Read the model definition and answer for the solid it produces. Units are mm, in the model's axes. Coordinates: 2 decimals unless noted, no trailing zeros. Loops run counter-clockwise (first coordinate to the right, second up) from the corner with the lowest first, then second, coordinate; pieces in that order, holes last. Notation, with made-up numbers: M -26.5,77 L -17.5,77 A5 cw -17.5,81 Z; hole C -26,63 d6. An arc over 180 degrees is marked long. One line per item, written item: value. Start each with the question number.
```python
from build123d import *

# Parameters (mm, degrees)
SKETCH1_W           = 120
SKETCH1_H           = 140
BOSS_EXTRUDE1_DEPTH = 3
SKETCH2_R           = 1.5
CUT_EXTRUDE1_DEPTH  = 107.343782141
SKETCH3_R           = 1.5
CUT_EXTRUDE3_DEPTH  = 107.343782141
SKETCH4_R           = 1.5
CUT_EXTRUDE4_DEPTH  = 107.343782141
SKETCH5_R           = 1.5
CUT_EXTRUDE5_DEPTH  = 3
SKETCH6_R           = 1.525
SKETCH6_W           = 10
SKETCH6_H           = 2.05
SKETCH6_W_2         = 20
CUT_EXTRUDE7_DEPTH  = 107.343782141
SKETCH9_R           = 1.525
CUT_EXTRUDE8_DEPTH  = 3
SKETCH10_W          = 50
SKETCH10_H          = 15
CUT_EXTRUDE9_DEPTH  = 5
SKETCH11_R          = 1.5
CUT_EXTRUDE10_DEPTH = 5
SKETCH12_W          = 2.05
SKETCH12_H          = 20
CUT_EXTRUDE11_DEPTH = 10


with BuildPart() as part:
    # Sketch1 → Boss-Extrude1 (new body)
    with BuildSketch(Plane(origin=(0, 0, 0), x_dir=(1, 0, 0), z_dir=(0, 1, 0))):
        Rectangle(SKETCH1_W, SKETCH1_H)
        Polygon((-80, 21.791828604), (-60, 10), (-60, 70), (-80, 70), align=None)
        Polygon((80, 70), (60, 70), (60, 10), (80, 21.791828604), align=None)
    extrude(amount=BOSS_EXTRUDE1_DEPTH)

    # Sketch2 → Cut-Extrude1 (cut, through all)
    with BuildSketch(Plane(origin=(0, 3, 0), x_dir=(1, 0, 0), z_dir=(0, 1, 0))):
        with Locations(Location((28, -60, 0), (0, 0, 270))):
            Circle(SKETCH2_R)
        with Locations(Location((40.6, -26.277010809, 0), (0, 0, 270))):
            Circle(SKETCH2_R)
        with Locations(Location((-50, -55, 0), (0, 0, 270))):
            Circle(SKETCH2_R)
        with Locations(Location((8, -55, 0), (0, 0, 270))):
            Circle(SKETCH2_R)
        with Locations(Location((-50, -28.6, 0), (0, 0, 270))):
            Circle(SKETCH2_R)
        with Locations(Location((8, -28.6, 0), (0, 0, 270))):
            Circle(SKETCH2_R)
    extrude(amount=-CUT_EXTRUDE1_DEPTH, mode=Mode.SUBTRACT)

    # Sketch3 → Cut-Extrude3 (cut, through all)
    with BuildSketch(Plane(origin=(0, 3, 0), x_dir=(1, 0, 0), z_dir=(0, 1, 0))):
        with Locations(Location((-26.529579069, 61.385555627, 0), (0, 0, 270))):
            Circle(SKETCH3_R)
        with Locations(Location((-26.529579069, 6.385555627, 0), (0, 0, 90))):
            Circle(SKETCH3_R)
        with Locations(Location((26.470420931, 6.385555627, 0), (0, 0, 270))):
            Circle(SKETCH3_R)
        with Locations(Location((26.470420931, 61.385555627, 0), (0, 0, 90))):
            Circle(SKETCH3_R)
    extrude(amount=-CUT_EXTRUDE3_DEPTH, mode=Mode.SUBTRACT)

    # Sketch4 → Cut-Extrude4 (cut, through all)
    with BuildSketch(Plane(origin=(0, 3, 0), x_dir=(1, 0, 0), z_dir=(0, 1, 0))):
        with Locations(Location((-75, 34.863883517, 0), (0, 0, 270))):
            Circle(SKETCH4_R)
        with Locations(Location((-75, 58.863883517, 0), (0, 0, 270))):
            Circle(SKETCH4_R)
        with Locations(Location((-46, 34.863883517, 0), (0, 0, 90))):
            Circle(SKETCH4_R)
        with Locations(Location((-46, 58.863883517, 0), (0, 0, 90))):
            Circle(SKETCH4_R)
        with Locations(Location((46, 58.863883517, 0), (0, 0, 270))):
            Circle(SKETCH4_R)
        with Locations(Location((46, 34.863883517, 0), (0, 0, 270))):
            Circle(SKETCH4_R)
        with Locations(Location((75, 34.863883517, 0), (0, 0, 90))):
            Circle(SKETCH4_R)
        with Locations(Location((75, 58.863883517, 0), (0, 0, 90))):
            Circle(SKETCH4_R)
    extrude(amount=-CUT_EXTRUDE4_DEPTH, mode=Mode.SUBTRACT)

    # Sketch5 → Cut-Extrude5 (cut)
    with BuildSketch(Plane(origin=(0, 3, 0), x_dir=(1, 0, 0), z_dir=(0, 1, 0))):
        with Locations(Location((-68, 30, 0), (0, 0, 270))):
            Circle(SKETCH5_R)
        with Locations(Location((-53, 30, 0), (0, 0, 270))):
            Circle(SKETCH5_R)
    extrude(amount=-CUT_EXTRUDE5_DEPTH, mode=Mode.SUBTRACT)

    # Sketch6 → Cut-Extrude7 (cut, through all)
    with BuildSketch(Plane(origin=(0, 3, 0), x_dir=(1, 0, 0), z_dir=(0, 1, 0))):
        with Locations(Location((-53, -64.8, 0), (0, 0, 270))):
            Circle(SKETCH6_R)
        with Locations(Location((53, -64.8, 0), (0, 0, 90))):
            Circle(SKETCH6_R)
        with Locations((-40, -53.975)):
            Rectangle(SKETCH6_W, SKETCH6_H)
        with Locations((40, -53.975)):
            Rectangle(SKETCH6_W, SKETCH6_H)
        with Locations((30, -21.725)):
            Rectangle(SKETCH6_W_2, SKETCH6_H)
        with Locations((-30, -21.725)):
            Rectangle(SKETCH6_W_2, SKETCH6_H)
        with Locations((35, 23.325)):
            Rectangle(SKETCH6_W, SKETCH6_H)
        with Locations((-35, 23.325)):
            Rectangle(SKETCH6_W, SKETCH6_H)
    extrude(amount=-CUT_EXTRUDE7_DEPTH, mode=Mode.SUBTRACT)

    # Sketch9 → Cut-Extrude8 (cut)
    with BuildSketch(Plane(origin=(0, 3, 0), x_dir=(1, 0, 0), z_dir=(0, 1, 0))):
        with Locations(Location((-54, 22, 0), (0, 0, 270))):
            Circle(SKETCH9_R)
        with Locations(Location((54, 22, 0), (0, 0, 90))):
            Circle(SKETCH9_R)
    extrude(amount=-CUT_EXTRUDE8_DEPTH, mode=Mode.SUBTRACT)

    # Sketch10 → Cut-Extrude9 (cut)
    with BuildSketch(Plane(origin=(0, 3, 0), x_dir=(1, 0, 0), z_dir=(0, 1, 0))):
        with Locations((-0.2, -8.475074484)):
            Rectangle(SKETCH10_W, SKETCH10_H)
    extrude(amount=-CUT_EXTRUDE9_DEPTH, mode=Mode.SUBTRACT)

    # Sketch11 → Cut-Extrude10 (cut)
    with BuildSketch(Plane(origin=(0, 3, 0), x_dir=(1, 0, 0), z_dir=(0, 1, 0))):
        with Locations(Location((-53, 64, 0), (0, 0, 270))):
            Circle(SKETCH11_R)
        with Locations(Location((53, 64, 0), (0, 0, 270))):
            Circle(SKETCH11_R)
    extrude(amount=-CUT_EXTRUDE10_DEPTH, mode=Mode.SUBTRACT)

    # Sketch12 → Cut-Extrude11 (cut)
    with BuildSketch(Plane(origin=(0, 3, 0), x_dir=(1, 0, 0), z_dir=(0, 1, 0))):
        with Locations((-55.975, -15)):
            Rectangle(SKETCH12_W, SKETCH12_H)
        with Locations((55.975, -15)):
            Rectangle(SKETCH12_W, SKETCH12_H)
    extrude(amount=-CUT_EXTRUDE11_DEPTH, mode=Mode.SUBTRACT)


solid = part.part
```
1) Flat-ended cylindrical pins translate along their axes: pin 1 (1.5 mm diameter, centred on y = 2, z = 12, fed in from +X); pin 2 (2.5 mm diameter, centred on x = 28, z = 60, fed in from +Y). Find the tip coordinate at first contact, or state that the pin passes through.
2) Consider line 1 along X through (y, z) = (0.3, -6.5); line 2 along X through (y, z) = (1.5, -30); line 3 along Z through (x, y) = (-46, 0.85). Determine where each line is inside the solid, lowest interval first.
3) Section B-B (y = 1.4) is taken. Count the separate pieces of the cut face and the enclosed holes in it, then the cut area to 3 significant figures.
4) Section A-A (x = -9.5) is taken. Determine the outline of the cut face in (y, z).
Results found:
1. pin 1: stops at x = 60
1. pin 2: passes through
2. line 1: x = -60 to -28.03, -25.03 to 24.97, 27.97 to 60
2. line 2: x = -80 to -69.5, -66.5 to -54.5, -51.5 to 80
2. line 3: z = -70 to -60.36, -57.36 to -36.36, -33.36 to 70
3. separate pieces: 1
3. enclosed holes: 35
3. area: 17,800 mm²
4. outline: M 0,-70 L 3,-70 L 3,0.98 L 0,0.98 Z; M 0,15.98 L 3,15.98 L 3,70 L 0,70 Z
